Check sheet for the modelled part. Datum: model origin and axes. Units: mm. Face numbers are marked on the shaded views. A direction names the side the tool comes from. Coordinates: 2 decimals unless noted, no trailing zeros. Order: outer loops, then holes, each group sorted by start corner. A loop starts at its lowest first (then second) coordinate and runs counter-clockwise, first axis right, second up.
1. Gauge pin test, flat ends, axial feed: pin 1 Ø12.5 at (y, z) = (28, -25) entering from +X; pin 2 Ø3.5 at (x, z) = (5, -45) entering from +Y; pin 3 Ø10 at (y, z) = (22, -16) entering from -X; pin 4 Ø10 at (x, y) = (44.5, 30.5) entering from -Z. Record the tip position at first contact, or that the pin passes through.
2. Cross-section at D-D (z = -25). Enter the section's corners in (x, y).
3. Thickness scan on line 1 (X direction, y = 1.7, z = -5); line 2 (Y direction, x = 27, z = -23); line 3 (Y direction, x = 45.25, z = -25). Record the ranges inside material, lowest first.
4. Set-up check for the marked faces 1, 2 and 3: record each of +Z, -Z, +X, -X, +Y, -Y from which the full face is reachable in a straight line by a thin tool's end or side.
5. Cross-section at A-A (z = -5). Enter the section's corners in (x, y), then the cut area to 3 significant figures.
6. Cross-section at B-B (x = 35). Enter the section's corners in (y, z), then the cut area to 3 significant figures.
7. Cross-section at C-C (y = 28). Enter the section's corners in (x, z).
8. Draft check along Y on the marked faces 4, 5, 6 and 7. Enter one of: released by +Y, released by -Y, zero draft, split by the parting line, or undercut.
```python
from build123d import *

# Parameters (mm, degrees)
ESQUISSE1_W             = 50
ESQUISSE1_H             = 50
BOSS_EXTRU_1_DEPTH      = 3
ESQUISSE2_W             = 9
ESQUISSE2_H             = 30
BOSS_EXTRU_2_DEPTH      = 47
ESQUISSE3_R             = 7
ENL_V_MAT_EXTRU_2_DEPTH = 3
ENL_V_MAT_EXTRU_3_REACH = 86.906
ESQUISSE4_R             = 10.75
CONG_1_R                = 10
ENL_V_MAT_EXTRU_4_REACH = 86.906
ESQUISSE5_R             = 1.5


with BuildPart() as part:
    # Esquisse1 → Boss.-Extru.1 (new body)
    with BuildSketch(Plane(origin=(0, 0, 0), x_dir=(1, 0, 0), z_dir=(0, 1, 0))):
        with Locations((25, 25)):
            Rectangle(ESQUISSE1_W, ESQUISSE1_H)
    extrude(amount=BOSS_EXTRU_1_DEPTH)

    # Esquisse2 → Boss.-Extru.2 (add)
    with BuildSketch(Plane(origin=(0, 3, 0), x_dir=(1, 0, 0), z_dir=(0, 1, 0))):
        with Locations((45.5, 25)):
            Rectangle(ESQUISSE2_W, ESQUISSE2_H)
    extrude(amount=BOSS_EXTRU_2_DEPTH)

    # Esquisse3 → Enlèv. mat.-Extru.2 (cut)
    with BuildSketch(Plane(origin=(50, 0, 0), x_dir=(0, 0, -1), z_dir=(1, 0, 0))):
        with Locations((25, 28)):
            Circle(ESQUISSE3_R)
    extrude(amount=-ENL_V_MAT_EXTRU_2_DEPTH, mode=Mode.SUBTRACT)

    # Esquisse4 → Enlèv. mat.-Extru.3 (cut, up to next)
    with BuildSketch(Plane(origin=(47, 0, 0), x_dir=(0, 0, -1), z_dir=(1, 0, 0)), mode=Mode.PRIVATE) as enl_v_mat_extru_3_sk1:
        with Locations((25, 28)):
            Circle(ESQUISSE4_R)
    enl_v_mat_extru_3_tool1 = extrude(enl_v_mat_extru_3_sk1.sketch, amount=-ENL_V_MAT_EXTRU_3_REACH, mode=Mode.PRIVATE) & part.part
    add(enl_v_mat_extru_3_tool1.solids().sort_by_distance((47, 28, -25))[0], mode=Mode.SUBTRACT)

    # Congé1
    cong_1_edges = [part.edges().sort_by_distance(p)[0] for p in [
        (45.5, 50, -40),
        (45.5, 50, -10),
    ]]
    fillet(cong_1_edges, radius=CONG_1_R)

    # Esquisse5 → Enlèv. mat.-Extru.4 (cut, up to next)
    with BuildSketch(Plane(origin=(0, 3, 0), x_dir=(1, 0, 0), z_dir=(0, 1, 0)), mode=Mode.PRIVATE) as enl_v_mat_extru_4_sk1:
        with Locations(Location((35, 45, 0), (0, 0, 270))):
            Circle(ESQUISSE5_R)
    enl_v_mat_extru_4_tool1 = extrude(enl_v_mat_extru_4_sk1.sketch, amount=-ENL_V_MAT_EXTRU_4_REACH, mode=Mode.PRIVATE) & part.part
    # Esquisse5 → Enlèv. mat.-Extru.4 (cut, up to next)
    with BuildSketch(Plane(origin=(0, 3, 0), x_dir=(1, 0, 0), z_dir=(0, 1, 0)), mode=Mode.PRIVATE) as enl_v_mat_extru_4_sk2:
        with Locations(Location((5, 45, 0), (0, 0, 270))):
            Circle(ESQUISSE5_R)
    enl_v_mat_extru_4_tool2 = extrude(enl_v_mat_extru_4_sk2.sketch, amount=-ENL_V_MAT_EXTRU_4_REACH, mode=Mode.PRIVATE) & part.part
    # Esquisse5 → Enlèv. mat.-Extru.4 (cut, up to next)
    with BuildSketch(Plane(origin=(0, 3, 0), x_dir=(1, 0, 0), z_dir=(0, 1, 0)), mode=Mode.PRIVATE) as enl_v_mat_extru_4_sk3:
        with Locations(Location((5, 5, 0), (0, 0, 270))):
            Circle(ESQUISSE5_R)
    enl_v_mat_extru_4_tool3 = extrude(enl_v_mat_extru_4_sk3.sketch, amount=-ENL_V_MAT_EXTRU_4_REACH, mode=Mode.PRIVATE) & part.part
    # Esquisse5 → Enlèv. mat.-Extru.4 (cut, up to next)
    with BuildSketch(Plane(origin=(0, 3, 0), x_dir=(1, 0, 0), z_dir=(0, 1, 0)), mode=Mode.PRIVATE) as enl_v_mat_extru_4_sk4:
        with Locations(Location((35, 5, 0), (0, 0, 270))):
            Circle(ESQUISSE5_R)
    enl_v_mat_extru_4_tool4 = extrude(enl_v_mat_extru_4_sk4.sketch, amount=-ENL_V_MAT_EXTRU_4_REACH, mode=Mode.PRIVATE) & part.part
    add(enl_v_mat_extru_4_tool1.solids().sort_by_distance((35, 3, -45))[0], mode=Mode.SUBTRACT)
    add(enl_v_mat_extru_4_tool2.solids().sort_by_distance((5, 3, -45))[0], mode=Mode.SUBTRACT)
    add(enl_v_mat_extru_4_tool3.solids().sort_by_distance((5, 3, -5))[0], mode=Mode.SUBTRACT)
    add(enl_v_mat_extru_4_tool4.solids().sort_by_distance((35, 3, -5))[0], mode=Mode.SUBTRACT)


solid = part.part
```
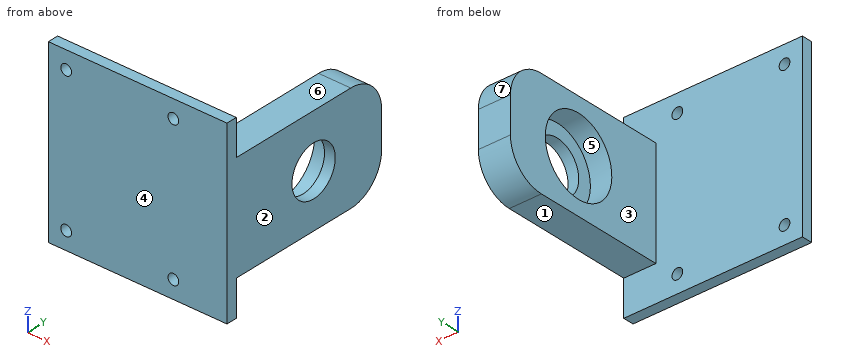
Data:
1. pin 1: passes through
1. pin 2: stops at y = 3
1. pin 3: stops at x = 41
1. pin 4: stops at z = -40
2. outline: (0, 0) - (50, 0) - (50, 21) - (47, 21) - (47, 17.25) - (41, 17.25) - (41, 3) - (0, 3) - close; (41, 38.75) - (47, 38.75) - (47, 35) - (50, 35) - (50, 50) - (41, 50) - close
3. line 1: x = 0 to 3.5, 6.5 to 33.5, 36.5 to 50
3. line 2: y = 0 to 3
3. line 3: y = 0 to 17.25, 38.75 to 50
4. face 1: -Z, +X, -X, +Y
4. face 2: +Z, -Z, +X, +Y, -Y
4. face 3: +Z, -Z, -X, +Y
5. outline: (0, 0) - (3.5, 0) - (3.5, 3) - (0, 3) - close; (6.5, 0) - (33.5, 0) - (33.5, 3) - (6.5, 3) - close; (36.5, 0) - (50, 0) - (50, 3) - (36.5, 3) - close
5. area: 132 mm2
6. outline: (0, -50) - (3, -50) - (3, -46.5) - (0, -46.5) - close; (0, -43.5) - (3, -43.5) - (3, -6.5) - (0, -6.5) - close; (0, -3.5) - (3, -3.5) - (3, 0) - (0, 0) - close
6. area: 132 mm2
7. outline: (41, -40) - (50, -40) - (50, -32) - (47, -32) - (47, -35.75) - (41, -35.75) - close; (41, -14.25) - (47, -14.25) - (47, -18) - (50, -18) - (50, -10) - (41, -10) - close
8. face 4: released by -Y
8. face 5: undercut
8. face 6: zero draft
8. face 7: released by +Y
